Check sheet for the modelled part. Datum: model origin and axes. Units: mm. Face numbers are marked on the shaded views. A direction names the side the tool comes from. Coordinates: 2 decimals unless noted, no trailing zeros. Order: outer loops, then holes, each group sorted by start corner. A loop starts at its lowest first (then second) coordinate and runs counter-clockwise, first axis right, second up. Notation, with made-up numbers: M 52.25,47 L 75.25,47 A7 ccw 75.25,60 Z; hole C -21,31 d6. An arc over 180 degrees is marked long. Answer in a Markdown table with one row per item. Add a question column.
from build123d import *

# Parameters (mm, degrees)
CYLINDER972_R     = 8.75
CYLINDER972_DEPTH = 4.2
CYLINDER973_R     = 4.45
CYLINDER973_DEPTH = 3.5
CHAMFER008_SIZE   = 3.5


with BuildPart() as cylinder1035:
    # Cylinder972 → Cylinder972 (new body)
    with BuildSketch(Plane.XY):
        Circle(CYLINDER972_R)
    extrude(amount=CYLINDER972_DEPTH)


with BuildPart() as planetary_gear:
    # Cylinder973 → Cylinder973 (new body)
    with BuildSketch(Plane.XY.offset(-3.5)):
        Circle(CYLINDER973_R)
    extrude(amount=CYLINDER973_DEPTH)

    # Fusion111: union Cylinder1035
    add(cylinder1035.part)

    # Chamfer008
    chamfer008_edges = [planetary_gear.edges().sort_by_distance(p)[0] for p in [
        (-8.75, 0, 4.2),
    ]]
    chamfer(chamfer008_edges, length=CHAMFER008_SIZE)


solid = planetary_gear.part
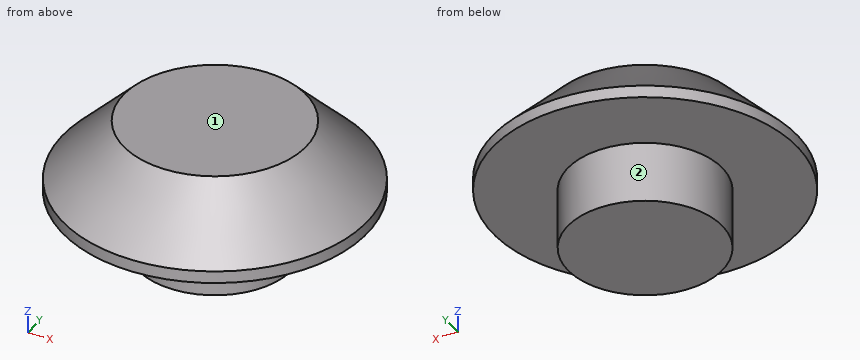
1. Scan lines: line 1 (Z direction, x = 4.75, y = 1.25); line 2 (X direction, y = 3, z = 3); line 3 (Z direction, x = 8, y = -1.75). Record each from-to range of solid material in increasing order.
2. Set-up check for the marked faces 1 and 2: record each of +Z, -Z, +X, -X, +Y, -Y from which the full face is reachable in a straight line by a thin tool's end or side.
3. Section check A-A on y = 0. Enter the section's corners in (x, z), then the cut area to 3 significant figures.
4. Go/stop test with flat-tipped pins: pin 1 Ø1 at (x, y) = (0.5, 6.5) entering from -Z; pin 2 Ø4 at (y, z) = (-6.5, 2) entering from +X. Record where each tip stops, or that it passes through.
5. Section check C-C on z = -2.25. Enter the section's corners in (x, y).
6. Section check D-D on z = 2.25. Enter the section's corners in (x, y).
Result sheet:
| question | item | result |
|---|---|---|
| 1 | line 1 | 0 to 4.2 |
| 1 | line 2 | -5.71 to 5.71 |
| 1 | line 3 | 0 to 1.26 |
| 2 | face 1 | +Z, +X, -X, +Y, -Y |
| 2 | face 2 | -Z |
| 3 | outline | M -8.75,0 L -4.45,0 L -4.45,-3.5 L 4.45,-3.5 L 4.45,0 L 8.75,0 L 8.75,0.7 L 5.25,4.2 L -5.25,4.2 L -8.75,0.7 Z |
| 3 | area | 92.4 mm^2 |
| 4 | pin 1 | z = 0 |
| 4 | pin 2 | x = 7.19 |
| 5 | outline | C 0,0 d8.9 |
| 6 | outline | C 0,0 d14.4 |
